```python
from build123d import *

# Parameters (mm, degrees)
SKETCH_1_R      = 4
EXTRUDE_1_DEPTH = 60


with BuildPart() as part:
    # 草图1 → 凸台-拉伸1 (new body)
    with BuildSketch(Plane(origin=(0, 0, 0), x_dir=(-1, 0, 0), z_dir=(0, 0, -1))):
        Polygon((3.464101615, -6), (6.92820323, 0), (3.464101615, 6), (-3.464101615, 6), (-6.92820323, 0), (-3.464101615, -6), align=None)
        Circle(SKETCH_1_R, mode=Mode.SUBTRACT)
    extrude(amount=-EXTRUDE_1_DEPTH)


solid = part.part
```
Geometry check sheet. Reference: the model listing, model coordinates, mm. Round coordinates to 2 decimals unless told otherwise and drop trailing zeros. Loops run counter-clockwise (first coordinate to the right, second up) from the corner with the lowest first, then second, coordinate; pieces in that order, holes last. Notation, with made-up numbers: (82, 59) - (102, 59) arc R21 ccw to (102, 86) - close; hole circle Ø3 at (11, 89). An arc over 180 degrees is marked (long way). Write each question's results on one line, items separated by ' | '. Start each with the question number.
Q1. Gauge pin test, flat ends, axial feed: P1, Ø4, axis at x = -5.5, z = 11, coming from the +Y side; P2, Ø1.5, axis at y = -2.5, z = 24.5, coming from the +X side. Record the tip position at first contact, or that the pin passes through.
Q2. Release check for a two-part mould opening along X. For faces 1 (the flat face through (-5.172, -3.042, 29.58)), 2 (the cylindrical face through (0.867, -3.905, 29.58)), 3 (the flat face through (5.172, 3.042, 29.58)) record: +X half, -X half, draft (parallel to the pull), parting line (faces both ways), or undercut.
Q3. Thickness scan on line 1 (Y direction, x = -2, z = 52.5); line 2 (Y direction, x = 0, z = 30); line 3 (X direction, y = -0.75, z = 7). Record the ranges inside material, lowest first. Write a range as [from, to].
Q4. Cross-section at D-D on x = -6. Enter the section's corners in (y, z).
Q5. Cross-section at B-B on y = 1.25. Enter the section's corners in (x, z).
Q6. Cross-section at C-C on z = 30.5. Enter the section's corners in (x, y).
Q7. Cross-section at A-A on x = 0. Enter the section's corners in (y, z), and give its area (3 significant figures).
Answers below:
1) P1: stops at y = 5.94 | P2: stops at x = 5.92
2) face 1: -X half | face 2: undercut | face 3: +X half
3) line 1: y = [-6, -3.46], [3.46, 6] | line 2: y = [-6, -4], [4, 6] | line 3: x = [-6.5, -3.93], [3.93, 6.5]
4) outline: (-1.61, 0) - (1.61, 0) - (1.61, 60) - (-1.61, 60) - close
5) outline: (-6.21, 0) - (-3.8, 0) - (-3.8, 60) - (-6.21, 60) - close; (3.8, 0) - (6.21, 0) - (6.21, 60) - (3.8, 60) - close
6) outline: (-6.93, 0) - (-3.46, -6) - (3.46, -6) - (6.93, 0) - (3.46, 6) - (-3.46, 6) - close; hole circle Ø8 at (0, 0)
7) outline: (-6, 0) - (-4, 0) - (-4, 60) - (-6, 60) - close; (4, 0) - (6, 0) - (6, 60) - (4, 60) - close | area: 240 mm²
